Model file for the job. Use its own axes, mm. A direction names the side the tool comes from. Round coordinates to 2 decimals unless told otherwise and drop trailing zeros. Order: outer loops, then holes, each group sorted by start corner. A loop starts at its lowest first (then second) coordinate and runs counter-clockwise, first axis right, second up. Notation, with made-up numbers: (10.5, 78) - (18.5, 78) arc R13 ccw to (18.5, 103) - close; hole circle Ø9 at (41.25, 6). An arc over 180 degrees is marked (long way). Write item = value, one per line.
```python
from build123d import *

# Parameters (mm, degrees)
F0_W          = 50.8
F0_H          = 50.8
F0_W_2        = 44.45
F0_H_2        = 44.45
F1_DEPTH      = 10
F1_DEPTH_BACK = 7
F3_D          = 5
F3_DEPTH      = 25.401
F4_D          = 5


# Not quite as in the source:
# - a feature names something its author has since deleted; it is built from what else it names


with BuildPart() as f1:
    # F0 (on Front) → F1 (new body, two sides)
    with BuildSketch(Plane.XZ) as f1_sk:
        Rectangle(F0_W, F0_H)
        Rectangle(F0_W_2, F0_H_2, mode=Mode.SUBTRACT)
    extrude(amount=F1_DEPTH)
    extrude(f1_sk.sketch, amount=-F1_DEPTH_BACK)

    # F3 (through all, one way)
    with BuildSketch(Plane(origin=(0, 0, 0), x_dir=(1, 0, 0), z_dir=(0, 0, -1))):
        with Locations((-10.4, 0), (10.2, 0)):
            Circle(F3_D / 2)
    extrude(amount=-F3_DEPTH, mode=Mode.SUBTRACT)

    # F4 (through all)
    with Locations(Plane.XY):
        with Locations((-10.4, 0), (10.2, 0)):
            Hole(F4_D / 2)


solid = f1.part
```
1) Cut at D-D (x = 10.2). Write the cut outline in (y, z) (3 decimals).
Conclusion:
outline = (-10, -25.4) - (-2.5, -25.4) - (-2.5, -22.225) - (-10, -22.225) - close; (-10, 22.225) - (-2.5, 22.225) - (-2.5, 25.4) - (-10, 25.4) - close; (2.5, -25.4) - (7, -25.4) - (7, -22.225) - (2.5, -22.225) - close; (2.5, 22.225) - (7, 22.225) - (7, 25.4) - (2.5, 25.4) - close
2) Wall check: line 1 along X through (y, z) = (-3.75, 10) (3 decimals); line 2 along Y through (x, z) = (10.2, -23.7). Give the ranges that are in metal, low to high.
Conclusion:
line_1 = -25.4 to -22.225, 22.225 to 25.4
line_2 = -10 to -2.5, 2.5 to 7
3) 3-axis set-ups, long thin cutter, end or side, ignore diameter. For faces 1 (the face through (0, -2, -22.225)), 2 (the face through (12.7, 0.1, -23.8)): which of +Z, -Z, +X, -X, +Y, -Y reach the whole face in a straight line?
Conclusion:
face_1 = +Y, -Y
face_2 = +Z, -Z
4) Cut at C-C (y = -6.25). Write the cut outline in (x, z) (3 decimals).
Conclusion:
outline = (-25.4, -25.4) - (25.4, -25.4) - (25.4, 25.4) - (-25.4, 25.4) - close; hole (-22.225, -22.225) - (22.225, -22.225) - (22.225, 22.225) - (-22.225, 22.225) - close
5) Mould opens along X. For faces 3 (the face through (-23, 7, 0)), 4 (the face through (-25.4, -2, 0)), 5 (the face through (-8.4, -1.5, -23.8)) say: +X half, -X half, draft (parallel to the pull), parting line (faces both ways), or undercut.
Conclusion:
face_3 = draft
face_4 = -X half
face_5 = undercut
6) Cut at B-B (x = -18). Write the cut outline in (y, z) (3 decimals).
Conclusion:
outline = (-10, -25.4) - (7, -25.4) - (7, -22.225) - (-10, -22.225) - close; (-10, 22.225) - (7, 22.225) - (7, 25.4) - (-10, 25.4) - close
7) Cut at A-A (z = -17.5). Write the cut outline in (x, y) (3 decimals).
Conclusion:
outline = (-25.4, -10) - (-22.225, -10) - (-22.225, 7) - (-25.4, 7) - close; (22.225, -10) - (25.4, -10) - (25.4, 7) - (22.225, 7) - close
